Design review of the part built by this model. Coordinates are the model's own, in mm. Face numbers are marked on the shaded views. Give positions to 0.01 mm unless a question says otherwise; leave off trailing zeros. Loops run counter-clockwise (first coordinate to the right, second up) from the corner with the lowest first, then second, coordinate; pieces in that order, holes last. Notation, with made-up numbers: (-15, 19) -> (33, 19) arc R24 cw to (33, 35) -> close; hole circle Ø2 at (6.25, 44.25). An arc over 180 degrees is marked (long way). Answer in a Markdown table with one row per item. Add a question column.
(1) Draft analysis for pull direction Y (two halves, no side actions). For the marked faces 1, 2 and 3, state which applies: +Y half, -Y half, draft (parallel to the pull), parting line (faces both ways), or undercut.
(2) For line 1 (Y direction, x = 0, z = 24.5); line 2 (Y direction, x = 3.5, z = 9.5); line 3 (X direction, y = -3, z = 11.5), list the stretches that pass through material, from the lowest coordinate up.
(3) For pin 1 (10 mm diameter, centred on x = -5, y = 5, fed in from -Z); pin 2 (3 mm diameter, centred on y = -4.5, z = 28, fed in from +X); pin 3 (4 mm diameter, centred on y = 4, z = 13, fed in from +X); pin 4 (3 mm diameter, centred on y = -6.5, z = 5, fed in from -X), all flat-tipped, find the tip position at first contact; note any pin that passes through.
(4) Consider section A-A on x = 0. Write out the cut boundary in (y, z), then the cut area to 3 significant figures.
(5) Consider section C-C on z = 4.5. Write out the cut boundary in (x, y), then the cut area to 3 significant figures.
from build123d import *

# Parameters (mm, degrees)
F0_R     = 10
F0_R_2   = 4.15
F1_DEPTH = 32
F2_SIZE  = 1
F3_SIZE  = 0.5


with BuildPart() as f1:
    # F0 (on Top) → F1 (new body)
    with BuildSketch(Plane.XY):
        Circle(F0_R)
        Circle(F0_R_2, mode=Mode.SUBTRACT)
    extrude(amount=F1_DEPTH)

    # F2
    f2_edges = [f1.edges().sort_by_distance(p)[0] for p in [
        (-10, 0, 32),
        (10, 0, 16),
        (-10, 0, 0),
    ]]
    chamfer(f2_edges, length=F2_SIZE)

    # F3
    f3_edges = [f1.edges().sort_by_distance(p)[0] for p in [
        (4.15, 0, 16),
        (-4.15, 0, 0),
        (-4.15, 0, 32),
    ]]
    chamfer(f3_edges, length=F3_SIZE)


solid = f1.part
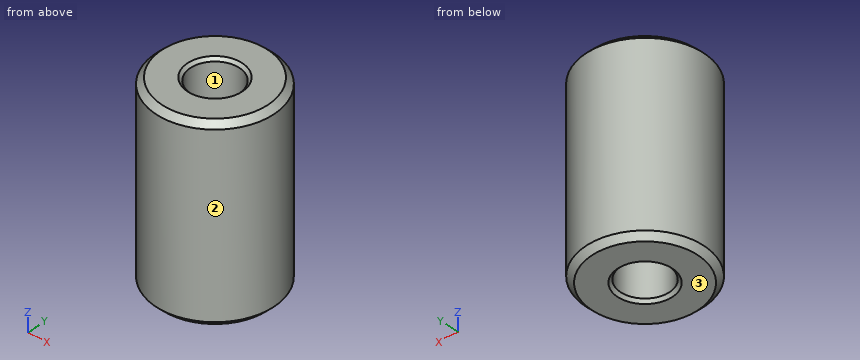
Values follow:
| question | item | result |
|---|---|---|
| 1 | face 1 | undercut |
| 1 | face 2 | parting line |
| 1 | face 3 | draft |
| 2 | line 1 | -10 to -4.15, 4.15 to 10 |
| 2 | line 2 | -9.37 to -2.23, 2.23 to 9.37 |
| 2 | line 3 | -9.54 to -2.87, 2.87 to 9.54 |
| 3 | pin 1 | z = 0 |
| 3 | pin 2 | x = 9.54 |
| 3 | pin 3 | x = 9.8 |
| 3 | pin 4 | x = -8.66 |
| 4 | outline | (-10, 1) -> (-9, 0) -> (-4.65, 0) -> (-4.15, 0.5) -> (-4.15, 31.5) -> (-4.65, 32) -> (-9, 32) -> (-10, 31) -> close; (4.15, 0.5) -> (4.65, 0) -> (9, 0) -> (10, 1) -> (10, 31) -> (9, 32) -> (4.65, 32) -> (4.15, 31.5) -> close |
| 4 | area | 372 mm2 |
| 5 | outline | circle Ø20 at (0, 0); hole circle Ø8.3 at (0, 0) |
| 5 | area | 260 mm2 |
